from build123d import *

# Parameters (mm, degrees)
F1_DEPTH = 6.1866333708
F2_R     = 3
F3_DEPTH = 2.4449569173
F4_DEPTH = 3.0221138149


with BuildPart() as f1:
    # F0 (on Top) → F1 (new body)
    with BuildSketch(Plane.XY):
        Polygon((8.3008821889, 36.7345147961), (0, 40.5132766051), (-8.3008821889, 36.7345147961), (-11.9557498605, 31.3451354549), (-11.9557498605, 24.7787649356), (-8.8584089335, 19.0796471245), (-2.9014659626, 22.3171101626), (-6.1513614195, 28.2969288261), (0, 33.5132766051), (6.1513614195, 28.2969288261), (2.9014659626, 22.3171101626), (8.8584089335, 19.0796471245), (11.9557498605, 24.7787649356), (11.9557498605, 31.3451354549), align=None)
    extrude(amount=F1_DEPTH)

    # F2
    f2_edges = [f1.edges().sort_by_distance(p)[0] for p in [
        (-11.95575, 24.778765, 3.093317),
        (0, 40.513277, 3.093317),
        (11.95575, 31.345135, 3.093317),
        (-11.95575, 31.345135, 3.093317),
        (6.151361, 28.296929, 3.093317),
        (8.300882, 36.734515, 3.093317),
        (-8.300882, 36.734515, 3.093317),
        (0, 33.513277, 3.093317),
        (11.95575, 24.778765, 3.093317),
        (-6.151361, 28.296929, 3.093317),
    ]]
    fillet(f2_edges, radius=F2_R)

    # F3 (add): a face of the model
    f3_faces = [f1.faces().sort_by_distance(p)[0] for p in [
        (5.879937448, 20.6983786435, 3.0933166854),
    ]]
    extrude(f3_faces, amount=F3_DEPTH)

    # F4 (add): a face of the model
    f4_faces = [f1.faces().sort_by_distance(p)[0] for p in [
        (-5.879937448, 20.6983786435, 3.0933166854),
    ]]
    extrude(f4_faces, amount=F4_DEPTH)


solid = f1.part
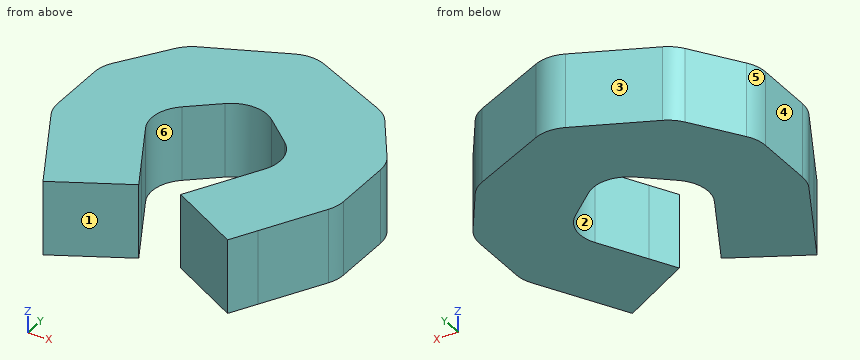
Read the model definition and answer for the solid it produces. Units are mm, in the model's axes. Face numbers are marked on the shaded views. A direction names the side the tool comes from. Coordinates: 2 decimals unless noted, no trailing zeros. Loops run counter-clockwise (first coordinate to the right, second up) from the corner with the lowest first, then second, coordinate; pieces in that order, holes last.
Q1. The part is cut by section A-A on y = 28.25. Write down the section's boundary in (x, z).
Q2. The part is cut by section B-B on z = 5.5. Write down the section's boundary in (x, y).
Q3. This flat-tipped pin is pushed along its axis until it touches: pin 1 Ø1 at (x, z) = (-4, 3) entering from +Y. Where does it stop, or does it pass through?
Q4. Which of the six approach directions +Z, -Z, +X, -X, +Y, -Y give full straight-line access (tool end or side, diameter ignored) to the marked faces 1, 2 and 3?
Q5. The part is cut by section D-D on x = 6. Write down the section's boundary in (y, z), and give its area (3 significant figures).
Q6. The mould has two halves that part along Y. Classify the marked faces 4, 5 and 6: +Y half, -Y half, draft (parallel to the pull), parting line (faces both ways), or undercut.
Q7. The part is cut by section C-C on y = 21. Write down the section's boundary in (x, z), and give its area (3 significant figures).
Q8. Consider probe 1 along X at (y, z) = (23.5, 3.75); probe 2 along X at (y, z) = (31.75, 1.75); probe 3 along Y at (x, z) = (-3.25, 3.75). Determine where each line is inside the solid, lowest interval first.
Results below:
1. outline: (-11.96, 0) - (-5.28, 0) - (-5.28, 6.19) - (-11.96, 6.19) - close; (5.28, 0) - (11.96, 0) - (11.96, 6.19) - (5.28, 6.19) - close
2. outline: (-11.96, 25.54) arc R3 ccw to (-11.59, 24.11) - (-7.42, 16.42) - (-1.46, 19.66) - (-4.99, 26.15) arc R3 cw to (-4.29, 29.87) - (-1.94, 31.87) arc R3 cw to (1.94, 31.87) - (4.29, 29.87) arc R3 cw to (4.99, 26.15) - (1.73, 20.17) - (7.69, 16.93) - (11.59, 24.11) arc R3 ccw to (11.96, 25.54) - (11.96, 30.42) arc R3 ccw to (11.44, 32.11) - (8.77, 36.04) arc R3 ccw to (7.53, 37.08) - (1.24, 39.95) arc R3 ccw to (-1.24, 39.95) - (-7.53, 37.08) arc R3 ccw to (-8.77, 36.04) - (-11.44, 32.11) arc R3 ccw to (-11.96, 30.42) - close
3. pin 1: stops at y = 38.92
4. face 1: +Z, -Z, -Y
4. face 2: +Z, -Z
4. face 3: +Z, -Z, -X, +Y
5. outline: (17.85, 0) - (37.78, 0) - (37.78, 6.19) - (17.85, 6.19) - close
5. area: 123 mm2
6. face 4: draft
6. face 5: +Y half
6. face 6: undercut
7. outline: (-9.9, 0) - (-2.19, 0) - (-2.19, 6.19) - (-9.9, 6.19) - close; (2.19, 0) - (9.9, 0) - (9.9, 6.19) - (2.19, 6.19) - close
7. area: 95.5 mm2
8. probe 1: x = -11.26 to -3.54, 3.54 to 11.26
8. probe 2: x = -11.65 to -2.08, 2.08 to 11.65
8. probe 3: y = 18.69 to 22.96, 30.76 to 39.03
